from build123d import *

# Parameters (mm, degrees)
F0_W     = 76.2
F0_H     = 76.2
F1_DEPTH = 76.2
F3_D     = 25.4
F5_DEPTH = 76.2
F6_R     = 2.936929
F7_DEPTH = 76.2


with BuildPart() as f1:
    # F0 (on Right) → F1 (new body)
    with BuildSketch(Plane.YZ):
        with Locations((2.936929, 13.631745)):
            Rectangle(F0_W, F0_H)
    extrude(amount=F1_DEPTH)

    # F3 (through all)
    with Locations(Plane.XY.offset(51.731745)):
        with Locations((38.1, 0)):
            Hole(F3_D / 2)

    # F4 (on face) → F5 (join)
    with BuildSketch(Plane.XZ.offset(35.163071)):
        Polygon((31.147685, 32.728756), (45.052315, 10.038463), (57.75037, 33.425371), align=None)
    extrude(amount=F5_DEPTH)

    # F6 (on face) → F7 (join)
    with BuildSketch(Plane.YZ.offset(76.2)):
        with Locations((0, 29.268674)):
            Circle(F6_R)
    extrude(amount=F7_DEPTH)


solid = f1.part
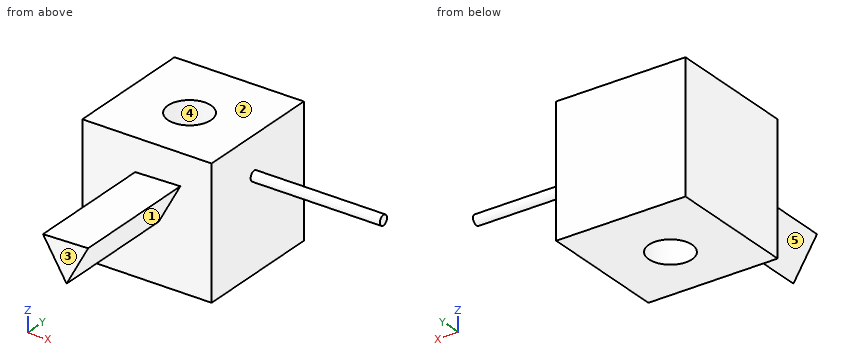
Verification items for the finished model (mm, model axes). Face numbers are marked on the shaded views. A direction names the side the tool comes from. Give positions to 0.01 mm unless a question says otherwise; leave off trailing zeros. Order: outer loops, then holes, each group sorted by start corner. A loop starts at its lowest first (then second) coordinate and runs counter-clockwise, first axis right, second up. Notation, with made-up numbers: M 13.25,-21.5 L 50.25,-21.5 A14 cw 50.25,-14.5 Z; hole C 27,-15.5 d6. An arc over 180 degrees is marked long. Use one line per item in the form item = value. Start each with the question number.
Q1. Section check D-D (y = -102). Enter the section's corners in (x, z).
Q2. Section check A-A (y = 0). Enter the section's corners in (x, z).
Q3. Access from +Z, -Z, +X, -X, +Y, -Y to the whole of each face (thin tool, end or side, straight path). Record for the marked faces 1 and 2.
Q4. Section check C-C (z = 41.5). Enter the section's corners in (x, y), then the cut area to 3 significant figures.
Q5. Go/stop test with a flat-tipped pin: pin 1 Ø12 at (x, z) = (116, 40.5) entering from +Y. Record where the tip stops, or that it passes through.
Q6. Section check B-B (x = 37). Enter the section's corners in (y, z).
Q7. Scan lines: line 1 along Y through (x, z) = (38, 15); line 2 along Y through (x, z) = (38, 32); line 3 along X through (y, z) = (-18, 2.5). Record each from-to range of solid material in increasing order. Write a range as [from, to].
Q8. Mould release check, pull along Y, two halves, no side actions. Record for the marked faces 3, 4 and 5: +Y half, -Y half, draft (parallel to the pull), parting line (faces both ways), or undercut.
Evaluation:
q1.outline = M 31.15,32.73 L 45.05,10.04 L 57.75,33.43 Z
q2.outline = M 0,-24.47 L 25.4,-24.47 L 25.4,51.73 L 0,51.73 Z; M 50.8,-24.47 L 76.2,-24.47 L 76.2,26.33 L 152.4,26.33 L 152.4,32.21 L 76.2,32.21 L 76.2,51.73 L 50.8,51.73 Z
q3.face_1 = -Z, +X, -Y
q3.face_2 = +Z, +X, -X, +Y, -Y
q4.outline = M 0,-35.16 L 76.2,-35.16 L 76.2,41.04 L 0,41.04 Z; hole C 38.1,0 d25.4
q4.area = 5,300 mm2
q5.pin_1 = through
q6.outline = M -111.36,23.18 L -35.16,23.18 L -35.16,-24.47 L -12.65,-24.47 L -12.65,51.73 L -35.16,51.73 L -35.16,32.88 L -111.36,32.88 Z; M 12.65,-24.47 L 41.04,-24.47 L 41.04,51.73 L 12.65,51.73 Z
q7.line_1 = [-35.16, -12.7], [12.7, 41.04]
q7.line_2 = [-111.36, -12.7], [12.7, 41.04]
q7.line_3 = [0, 76.2]
q8.face_3 = -Y half
q8.face_4 = undercut
q8.face_5 = draft
